Input: part model. Units: mm. Frame: model coordinates. A direction names the side the tool comes from. Give positions to 0.01 mm unless a question says otherwise; leave off trailing zeros. Loops run counter-clockwise (first coordinate to the right, second up) from the corner with the lowest first, then second, coordinate; pieces in that order, holes last.
from build123d import *

# Parameters (mm, degrees)
SKETCH1_W           = 328.676
SKETCH1_H           = 100.076
SKETCH1_W_2         = 327.152
SKETCH1_H_2         = 98.552
SKETCH1_W_3         = 323.977
SKETCH1_H_3         = 95.377
SKETCH1_W_4         = 318.897
SKETCH1_H_4         = 90.297
BOSS_EXTRUDE1_DEPTH = 2.54
SKETCH1_3_W         = 328.676
SKETCH1_3_H         = 100.076
SKETCH1_3_W_2       = 327.152
SKETCH1_3_H_2       = 98.552
BOSS_EXTRUDE2_DEPTH = 12.065
SKETCH1_4_W         = 327.152
SKETCH1_4_H         = 98.552
SKETCH1_4_W_2       = 323.977
SKETCH1_4_H_2       = 95.377
BOSS_EXTRUDE3_DEPTH = 10.3505
SKETCH1_5_W         = 323.977
SKETCH1_5_H         = 95.377
SKETCH1_5_W_2       = 318.897
SKETCH1_5_H_2       = 90.297
BOSS_EXTRUDE4_DEPTH = 6.8072
FILLET1_R           = 4.7625
SKETCH2_R           = 2.8575
SKETCH2_R_2         = 1.35255
BOSS_EXTRUDE5_DEPTH = 4.2672


with BuildPart() as part:
    # Sketch1 → Boss-Extrude1 (new body)
    # profile 1 of 4: a face of its own
    with BuildSketch(Plane.XY):
        Rectangle(SKETCH1_W, SKETCH1_H)
        Rectangle(SKETCH1_W_2, SKETCH1_H_2, mode=Mode.SUBTRACT)
    # profile 2 of 4: a face of its own
    with BuildSketch(Plane.XY):
        Rectangle(SKETCH1_W_2, SKETCH1_H_2)
        Rectangle(SKETCH1_W_3, SKETCH1_H_3, mode=Mode.SUBTRACT)
    # profile 3 of 4: a face of its own
    with BuildSketch(Plane.XY):
        Rectangle(SKETCH1_W_3, SKETCH1_H_3)
    # profile 4 of 4: a face of its own
    with BuildSketch(Plane.XY):
        Rectangle(SKETCH1_W_4, SKETCH1_H_4)
    extrude(amount=BOSS_EXTRUDE1_DEPTH)

    # Sketch1<3> → Boss-Extrude2 (add)
    with BuildSketch(Plane.XY):
        Rectangle(SKETCH1_3_W, SKETCH1_3_H)
        Rectangle(SKETCH1_3_W_2, SKETCH1_3_H_2, mode=Mode.SUBTRACT)
    extrude(amount=BOSS_EXTRUDE2_DEPTH)

    # Sketch1<4> → Boss-Extrude3 (add)
    with BuildSketch(Plane.XY):
        Rectangle(SKETCH1_4_W, SKETCH1_4_H)
        Rectangle(SKETCH1_4_W_2, SKETCH1_4_H_2, mode=Mode.SUBTRACT)
    extrude(amount=BOSS_EXTRUDE3_DEPTH)

    # Sketch1<5> → Boss-Extrude4 (add)
    with BuildSketch(Plane.XY):
        Rectangle(SKETCH1_5_W, SKETCH1_5_H)
        Rectangle(SKETCH1_5_W_2, SKETCH1_5_H_2, mode=Mode.SUBTRACT)
    extrude(amount=BOSS_EXTRUDE4_DEPTH)

    # Fillet1
    fillet1_edges = [part.edges().sort_by_distance(p)[0] for p in [
        (159.4485, 45.1485, 4.6736),
        (159.4485, -45.1485, 4.6736),
        (-159.4485, -45.1485, 4.6736),
        (-159.4485, 45.1485, 4.6736),
        (163.576, -49.276, 11.20775),
        (-163.576, -49.276, 11.20775),
        (-163.576, 49.276, 11.20775),
        (163.576, 49.276, 11.20775),
        (161.9885, 47.6885, 8.57885),
        (-161.9885, 47.6885, 8.57885),
        (-161.9885, -47.6885, 8.57885),
        (161.9885, -47.6885, 8.57885),
    ]]
    fillet(fillet1_edges, radius=FILLET1_R)

    # Sketch2 → Boss-Extrude5 (add)
    # profile 1 of 6: a face of its own
    with BuildSketch(Plane.XY.offset(2.54)):
        with Locations((142.875, -28.575)):
            Circle(SKETCH2_R)
        with Locations((142.875, -28.575)):
            Circle(SKETCH2_R_2, mode=Mode.SUBTRACT)
    # profile 2 of 6: a face of its own
    with BuildSketch(Plane.XY.offset(2.54)):
        with Locations((142.875, 28.575)):
            Circle(SKETCH2_R)
        with Locations((142.875, 28.575)):
            Circle(SKETCH2_R_2, mode=Mode.SUBTRACT)
    # profile 3 of 6: a face of its own
    with BuildSketch(Plane.XY.offset(2.54)):
        with Locations((-42.8625, 0)):
            Circle(SKETCH2_R)
        with Locations((-42.8625, 0)):
            Circle(SKETCH2_R_2, mode=Mode.SUBTRACT)
    # profile 4 of 6: a face of its own
    with BuildSketch(Plane.XY.offset(2.54)):
        with Locations((33.3375, 0)):
            Circle(SKETCH2_R)
        with Locations((33.3375, 0)):
            Circle(SKETCH2_R_2, mode=Mode.SUBTRACT)
    # profile 5 of 6: a face of its own
    with BuildSketch(Plane.XY.offset(2.54)):
        with Locations((-142.875, 28.575)):
            Circle(SKETCH2_R)
        with Locations((-142.875, 28.575)):
            Circle(SKETCH2_R_2, mode=Mode.SUBTRACT)
    # profile 6 of 6: a face of its own
    with BuildSketch(Plane.XY.offset(2.54)):
        with Locations((-138.1125, -28.575)):
            Circle(SKETCH2_R)
        with Locations((-138.1125, -28.575)):
            Circle(SKETCH2_R_2, mode=Mode.SUBTRACT)
    extrude(amount=BOSS_EXTRUDE5_DEPTH)


solid = part.part
(1) Ray query, probe 1 along X at (y, z) = (22.5, 5.25); probe 2 along Y at (x, z) = (93, 8.5); probe 3 along X at (y, z) = (-25, 7). Return the intervals inside material, ascending.
Values follow:
probe 1: x = -164.34 to -159.45, 159.45 to 164.34
probe 2: y = -50.04 to -47.69, 47.69 to 50.04
probe 3: x = -164.34 to -161.99, 161.99 to 164.34
(2) Cut plane B-B (y = 21.5). Return the cut outline in (x, z) (1 decimal), and give its area (3 significant figures).
Values follow:
outline: (-164.3, 0) - (164.3, 0) - (164.3, 12.1) - (163.6, 12.1) - (163.6, 10.4) - (162, 10.4) - (162, 6.8) - (159.4, 6.8) - (159.4, 2.5) - (-159.4, 2.5) - (-159.4, 6.8) - (-162, 6.8) - (-162, 10.4) - (-163.6, 10.4) - (-163.6, 12.1) - (-164.3, 12.1) - close
area: 896 mm2
(3) Mould query, pull axis X, two halves, no side actions, for faces 1 (the flat face through (-2, -50.038, 6)), 2 (the cylindrical face through (145.515, 27.481, 4.644)), 3 (the flat face through (-164.338, -1, 6)). Classes: +X half, -X half, draft (parallel to the pull), parting line (faces both ways), or undercut.
Values follow:
face 1: draft
face 2: undercut
face 3: -X half
(4) Pin query (flat end, axial travel): pin 1 Ø3 at (x, y) = (-42.86, 0) entering from +Z; pin 2 Ø1.4 at (x, y) = (-138, -28) entering from +Z. Return the tip coordinate at first contact, or that it passes through.
Values follow:
pin 1: stops at z = 6.81
pin 2: stops at z = 2.54
(5) Cut plane A-A (x = 12). Return the cut outline in (y, z) (1 decimal), and give its area (3 significant figures).
Values follow:
outline: (-50, 0) - (50, 0) - (50, 12.1) - (49.3, 12.1) - (49.3, 10.4) - (47.7, 10.4) - (47.7, 6.8) - (45.1, 6.8) - (45.1, 2.5) - (-45.1, 2.5) - (-45.1, 6.8) - (-47.7, 6.8) - (-47.7, 10.4) - (-49.3, 10.4) - (-49.3, 12.1) - (-50, 12.1) - close
area: 315 mm2
(6) Reachability of faces 4 (the cylindrical face through (-140.235, 27.481, 4.644)), 5 (the flat face through (-2, 50.038, 6)) from +Z, -Z, +X, -X, +Y, -Y: full face, straight path, thin tool, end or side. Return the list, or none.
Values follow:
face 4: +Z
face 5: +Z, -Z, +X, -X, +Y
